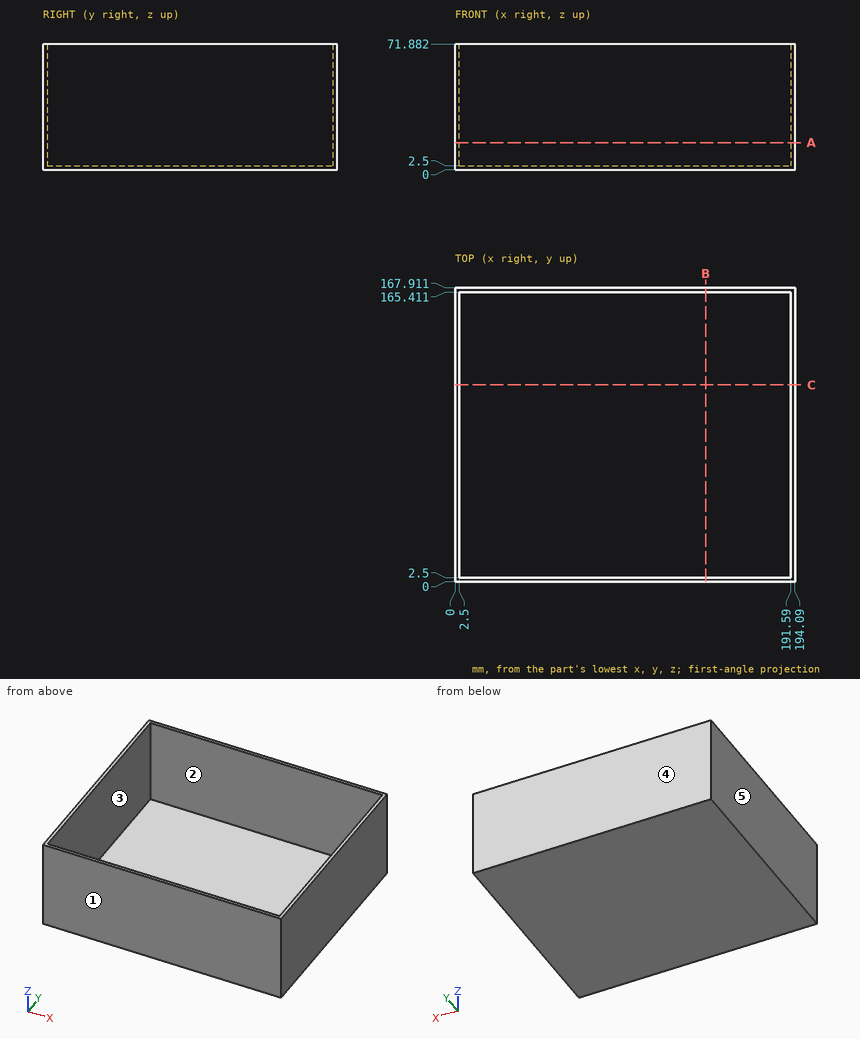
Could you check a few things on this drawing? It's one solid part, dimensions in mm from its lowest x, y, z. A direction names the side the tool comes from. Round coordinates to 2 decimals unless told otherwise and drop trailing zeros. Order: outer loops, then holes, each group sorted by start corner. A loop starts at its lowest first (then second) coordinate and runs counter-clockwise, first axis right, second up.
Q1. Imagine slicing it at A-A, the plane z = 15.5. List the corners of the cut face in (x, y) for me.
Geometry says:
outline: (0, 0) - (194.09, 0) - (194.09, 167.91) - (0, 167.91) - close; hole (2.5, 2.5) - (191.59, 2.5) - (191.59, 165.41) - (2.5, 165.41) - close
Q2. Imagine slicing it at B-B, the plane x = 143. List the corners of the cut face in (y, z) for me.
Geometry says:
outline: (0, 0) - (167.91, 0) - (167.91, 71.88) - (165.41, 71.88) - (165.41, 2.5) - (2.5, 2.5) - (2.5, 71.88) - (0, 71.88) - close
Q3. I'm going to push flat-ended pins straight in: P1, Ø1.5, axis at x = 86.5, y = 107.5, coming from the +Z side; P2, Ø10, axis at y = 149, z = 10.5, coming from the -X side. Where does each tip first touch, or does it pass through?
Geometry says:
P1: stops at z = 2.5
P2: stops at x = 0
Q4. Thinking about a two-plate mould opening in Y: for the marked faces 3, 4 and 5, which applies, released by +Y, released by -Y, zero draft, split by the parting line, or undercut?
Geometry says:
face 3: undercut
face 4: released by +Y
face 5: zero draft
Q5. Imagine slicing it at C-C, the plane y = 112.5. List the corners of the cut face in (x, z) for me, then the cut area to 3 significant figures.
Geometry says:
outline: (0, 0) - (194.09, 0) - (194.09, 71.88) - (191.59, 71.88) - (191.59, 2.5) - (2.5, 2.5) - (2.5, 71.88) - (0, 71.88) - close
area: 832 mm2
Q6. Which directions (+Z, -Z, +X, -X, +Y, -Y) give clear straight access to the entire face, cutting with the end or side of a thin tool? Please do the marked faces 1 and 2.
Geometry says:
face 1: +Z, -Z, +X, -X, -Y
face 2: +Z
Q7. Please list where these lines run through material, in increasing order: probe 1 along Y at (x, z) = (30, 7.5); probe 2 along X at (y, z) = (50, 54); probe 3 along Z at (x, y) = (128, 26).
Geometry says:
probe 1: y = 0 to 2.5, 165.41 to 167.91
probe 2: x = 0 to 2.5, 191.59 to 194.09
probe 3: z = 0 to 2.5
